The figure shows three views and two pictorial views of one solid part (mm, origin at its lowest corner). Answer the questions. A direction names the side the tool comes from. Coordinates: 2 decimals unless noted, no trailing zeros. Write each loop counter-clockwise with the first axis right and the second up, starting at its lowest first coordinate (ties: lowest second). Pieces come first, ordered by that corner, then holes.
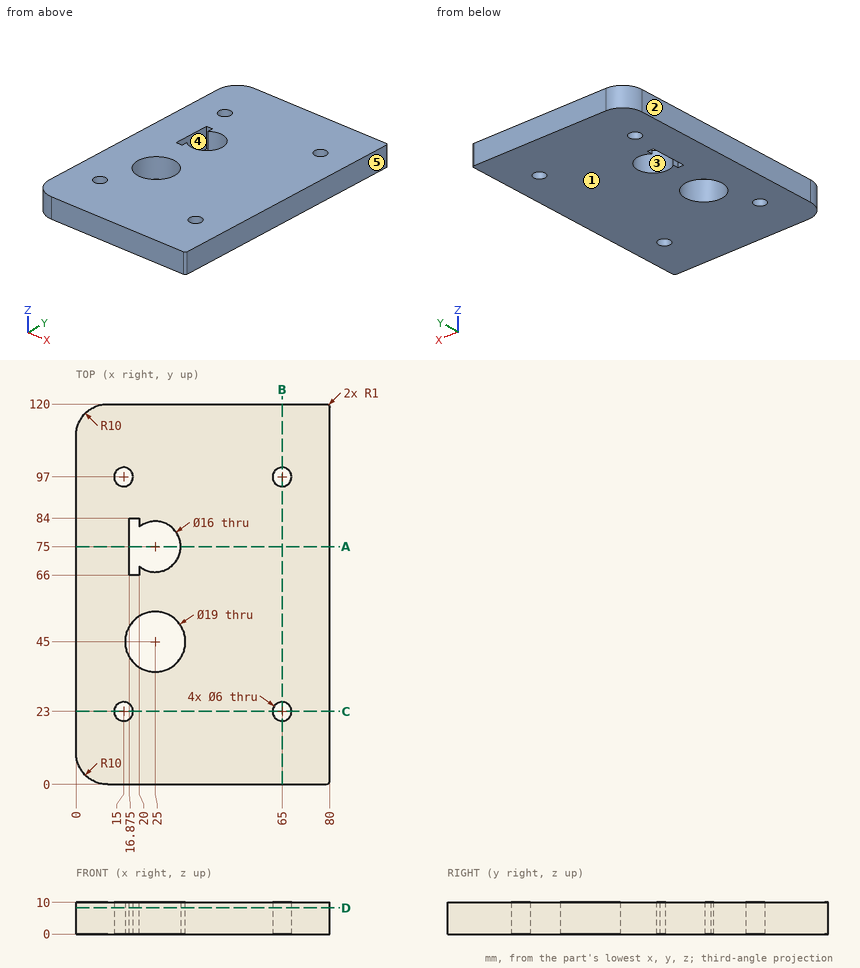
1. Section C-C on y = 23 is taken. Give the vertices of the cut face in (x, z).
Results found:
outline: (0, 0) - (12, 0) - (12, 10) - (0, 10) - close; (18, 0) - (62, 0) - (62, 10) - (18, 10) - close; (68, 0) - (80, 0) - (80, 10) - (68, 10) - close
2. Section A-A on y = 75 is taken. Give the vertices of the cut face in (x, z) (3 decimals).
Results found:
outline: (0, 0) - (16.875, 0) - (16.875, 10) - (0, 10) - close; (33, 0) - (80, 0) - (80, 10) - (33, 10) - close
3. For a pull along X with two mould halves and no side action, classify the marked faces 1, 2 and 3 as pulls with the +X half, pulls with the -X half, needs draft (parallel to the pull), parting line crosses it, or undercut.
Results found:
face 1: needs draft
face 2: pulls with the -X half
face 3: undercut
4. Section B-B on x = 65 is taken. Give the vertices of the cut face in (y, z).
Results found:
outline: (0, 0) - (20, 0) - (20, 10) - (0, 10) - close; (26, 0) - (94, 0) - (94, 10) - (26, 10) - close; (100, 0) - (120, 0) - (120, 10) - (100, 10) - close
5. A flat-ended cylindrical pin translates along its axis: P1, Ø15, axis at x = 25, y = 45, coming from the -Z side. Find the tip coordinate at first contact, or state that the pin passes through.
Results found:
P1: passes through
6. A tool of negligible diameter and unlimited length cuts with its end or side. For the marked faces 4 and 5, from which of +Z, -Z, +X, -X, +Y, -Y can it reach the whole face along a straight path? Write none if from no direction.
Results found:
face 4: +Z, -Z
face 5: +Z, -Z, +X, +Y, -Y
7. Find the intervals of material crossed by L1, parallel to Y at x = 15, z = 5; L2, parallel to Y at x = 13, z = 4.25; L3, parallel to X at y = 75, z = 2.75 (3 decimals), in increasing order.
Results found:
L1: y = 0 to 20, 26 to 94, 100 to 120
L2: y = 0 to 20.76, 25.24 to 94.76, 99.24 to 120
L3: x = 0 to 16.875, 33 to 80
8. Section D-D on z = 8.25 is taken. Give the vertices of the cut face in (x, y) (3 decimals), then the cut area to 3 significant figures.
Results found:
outline: (0, 10) arc R10 ccw to (10, 0) - (79, 0) arc R1 ccw to (80, 1) - (80, 119) arc R1 ccw to (79, 120) - (10, 120) arc R10 ccw to (0, 110) - close; hole circle Ø6 at (15, 23); hole circle Ø6 at (15, 97); hole circle Ø19 at (25, 45); hole (16.875, 66) - (20, 66) - (20, 68.755) arc R8 ccw (long way) to (20, 81.245) - (20, 84) - (16.875, 84) - close; hole circle Ø6 at (65, 23); hole circle Ø6 at (65, 97)
area: 8,930 mm2
